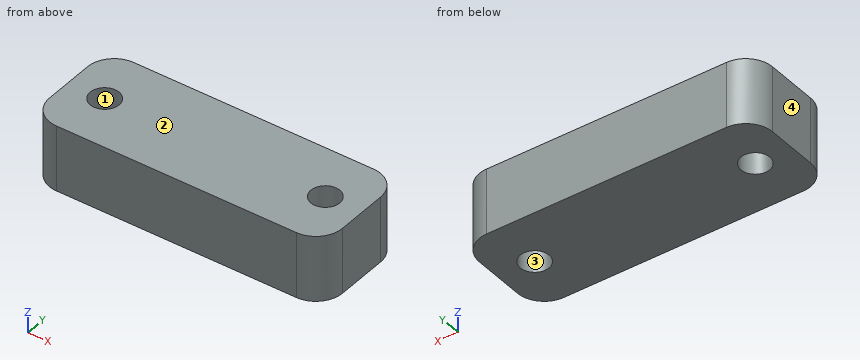
```python
from build123d import *

# Parameters (mm, degrees)
F0_W     = 55.8
F0_H     = 20
F1_DEPTH = 12.5
F2_D     = 5.5
F3_R     = 5.08


with BuildPart() as f1:
    # F0 (on Top) → F1 (new body)
    with BuildSketch(Plane.XY):
        Rectangle(F0_W, F0_H)
    extrude(amount=-F1_DEPTH)

    # F2 (through all)
    with Locations(Plane.XY):
        with Locations((21, 0), (-21, 0)):
            Hole(F2_D / 2)

    # F3
    f3_edges = [f1.edges().sort_by_distance(p)[0] for p in [
        (27.9, 10, -6.25),
        (27.9, -10, -6.25),
        (-27.9, -10, -6.25),
        (-27.9, 10, -6.25),
    ]]
    fillet(f3_edges, radius=F3_R)


solid = f1.part
```
Input: part model. Units: mm. Frame: model coordinates. Face numbers are marked on the shaded views. Coordinates: 2 decimals unless noted, no trailing zeros. Write each loop counter-clockwise with the first axis right and the second up, starting at its lowest first coordinate (ties: lowest second). Pieces come first, ordered by that corner, then holes. Notation, with made-up numbers: (52.5, 23.25) -> (62.5, 23.25) arc R16 ccw to (62.5, 53.25) -> close; hole circle Ø9 at (68.5, 89.25). An arc over 180 degrees is marked (long way). Answer as a JSON object with one key per item and string values.
1. Mould query, pull axis X, two halves, no side actions, for the marked faces 1, 2, 3 and 4. Classes: released by +X, released by -X, zero draft, split by the parting line, or undercut.
Result set:
{"face 1": "undercut", "face 2": "zero draft", "face 3": "undercut", "face 4": "released by -X"}
2. First-contact query: P1, Ø2, axis at y = -7, z = -8, coming from the +X side. Flat tip, straight axial feed; report the tip coordinate or a pass-through.
Result set:
{"P1": "stops at x = 27.78"}
3. Section B-B on y = 0. Return the cut outline in (x, z).
Result set:
{"outline": "(-27.9, -12.5) -> (-23.75, -12.5) -> (-23.75, 0) -> (-27.9, 0) -> close; (-18.25, -12.5) -> (18.25, -12.5) -> (18.25, 0) -> (-18.25, 0) -> close; (23.75, -12.5) -> (27.9, -12.5) -> (27.9, 0) -> (23.75, 0) -> close"}
4. Section A-A on x = -21. Return the cut outline in (y, z).
Result set:
{"outline": "(-10, -12.5) -> (-2.75, -12.5) -> (-2.75, 0) -> (-10, 0) -> close; (2.75, -12.5) -> (10, -12.5) -> (10, 0) -> (2.75, 0) -> close"}
5. Section D-D on y = -7. Return the cut outline in (x, z).
Result set:
{"outline": "(-27.45, -12.5) -> (27.45, -12.5) -> (27.45, 0) -> (-27.45, 0) -> close"}
6. Section C-C on z = -11.5. Return the cut outline in (x, y).
Result set:
{"outline": "(-27.9, -4.92) arc R5.08 ccw to (-22.82, -10) -> (22.82, -10) arc R5.08 ccw to (27.9, -4.92) -> (27.9, 4.92) arc R5.08 ccw to (22.82, 10) -> (-22.82, 10) arc R5.08 ccw to (-27.9, 4.92) -> close; hole circle Ø5.5 at (-21, 0); hole circle Ø5.5 at (21, 0)"}
7. Material intervals for line 1 (X direction, y = -0.25, z = -0.25); line 2 (Y direction, x = -21, z = -9.75); line 3 (X direction, y = 2, z = -1.25), sorted ascending. Write a range as from..to.
Result set:
{"line 1": "x = -27.9..-23.74, -18.26..18.26, 23.74..27.9", "line 2": "y = -10..-2.75, 2.75..10", "line 3": "x = -27.9..-22.89, -19.11..19.11, 22.89..27.9"}
